Part model, mm, in its own coordinate system. Face numbers are marked on the shaded views. A direction names the side the tool comes from. Coordinates: 2 decimals unless noted, no trailing zeros. Order: outer loops, then holes, each group sorted by start corner. A loop starts at its lowest first (then second) coordinate and runs counter-clockwise, first axis right, second up.
from build123d import *

# Parameters (mm, degrees)
SKICA1_R                 = 45
P_IDAT_VYSUNUT_M1_DEPTH  = 10
SKICA3_R                 = 5
ODEBRAT_VYSUNUT_M1_DEPTH = 65.420493634
KRUHOV_POLE1_COUNT       = 4
SKICA4_R                 = 20
P_IDAT_VYSUNUT_M2_DEPTH  = 50
SKICA5_R                 = 10
ODEBRAT_VYSUNUT_M2_DEPTH = 81.932070281
ZAOBLIT1_R               = 5
ZKOSEN_1_SIZE            = 5


with BuildPart() as part:
    # Skica1 → Přidat vysunutím1 (new body)
    with BuildSketch(Plane(origin=(0, 0, 0), x_dir=(1, 0, 0), z_dir=(0, 1, 0))):
        with Locations(Location((0, 0, 0), (0, 0, 270))):
            Circle(SKICA1_R)
    extrude(amount=P_IDAT_VYSUNUT_M1_DEPTH)

    # Skica3 → Odebrat vysunutím1 (cut, through all)
    with BuildSketch(Plane(origin=(0, 10, 0), x_dir=(1, 0, 0), z_dir=(0, 1, 0))):
        with Locations(Location((0, 35, 0), (0, 0, 270))):
            Circle(SKICA3_R)
    odebrat_vysunut_m1 = extrude(amount=-ODEBRAT_VYSUNUT_M1_DEPTH, mode=Mode.SUBTRACT)

    # Kruhové pole1: Odebrat vysunutím1 ×4 about axis
    kruhov_pole1_axis = Axis((0, 0, 0), (0, 1, 0))
    for i in range(1, KRUHOV_POLE1_COUNT):
        add(odebrat_vysunut_m1.rotate(kruhov_pole1_axis, i * 360 / KRUHOV_POLE1_COUNT), mode=Mode.SUBTRACT)

    # Skica4 → Přidat vysunutím2 (add)
    with BuildSketch(Plane(origin=(0, 10, 0), x_dir=(1, 0, 0), z_dir=(0, 1, 0))):
        with Locations(Location((0, 0, 0), (0, 0, 270))):
            Circle(SKICA4_R)
    extrude(amount=-P_IDAT_VYSUNUT_M2_DEPTH)

    # Skica5 → Odebrat vysunutím2 (cut, through all)
    with BuildSketch(Plane.XZ.offset(40)):
        with Locations(Location((0, 0, 0), (0, 0, 270))):
            Circle(SKICA5_R)
    extrude(amount=-ODEBRAT_VYSUNUT_M2_DEPTH, mode=Mode.SUBTRACT)

    # Zaoblit1
    zaoblit1_edges = [part.edges().sort_by_distance(p)[0] for p in [
        (0, 0, -20),
    ]]
    fillet(zaoblit1_edges, radius=ZAOBLIT1_R)

    # Zkosení1
    zkosen_1_edges = [part.edges().sort_by_distance(p)[0] for p in [
        (0, -40, -20),
    ]]
    chamfer(zkosen_1_edges, length=ZKOSEN_1_SIZE)


solid = part.part
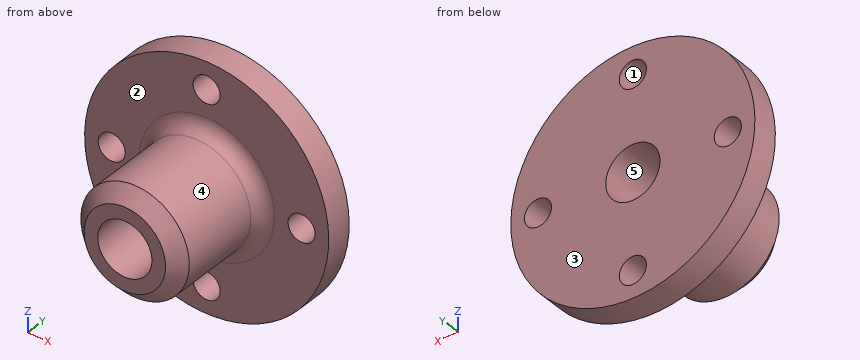
Q1. Which spindle directions (+Z, -Z, +X, -X, +Y, -Y) get a long thin tool onto all of the face, cutting with end or side? Do the marked faces 1 and 2. Say none if no direction does.
Results list:
face 1: +Y, -Y
face 2: -Y
Q2. Cut at B-B on z = 0. Write the cut outline in (x, y), and give its area (3 significant figures).
Results list:
outline: (-45, 0) - (-40, 0) - (-40, 10) - (-45, 10) - close; (-30, 0) - (-25, 0) arc R5 cw to (-20, -5) - (-20, -35) - (-15, -40) - (-10, -40) - (-10, 10) - (-30, 10) - close; (10, -40) - (15, -40) - (20, -35) - (20, -5) arc R5 cw to (25, 0) - (30, 0) - (30, 10) - (10, 10) - close; (40, 0) - (45, 0) - (45, 10) - (40, 10) - close
area: 1,290 mm2
Q3. Wall check: line 1 along X through (y, z) = (-27, 0); line 2 along Z through (x, y) = (0.5, -20); line 3 along Y through (x, z) = (27.5, -26.5). Give the ranges that are in metal, low to high.
Results list:
line 1: x = -20 to -10, 10 to 20
line 2: z = -19.99 to -9.99, 9.99 to 19.99
line 3: y = 0 to 10
Q4. Cut at C-C on z = 35. Write the cut outline in (x, y), and give its area (3 significant figures).
Results list:
outline: (-28.28, 0) - (-5, 0) - (-5, 10) - (-28.28, 10) - close; (5, 0) - (28.28, 0) - (28.28, 10) - (5, 10) - close
area: 466 mm2
Q5. Mould opens along Z. For the marked faces 3, 4 and 5 say: pulls with the +Z half, pulls with the -Z half, needs draft (parallel to the pull), parting line crosses it, or undercut.
Results list:
face 3: needs draft
face 4: parting line crosses it
face 5: undercut
Q6. Cut at A-A on x = 0. Write the cut outline in (y, z).
Results list:
outline: (-40, -15) - (-35, -20) - (-5, -20) arc R5 cw to (0, -25) - (0, -30) - (10, -30) - (10, -10) - (-40, -10) - close; (-40, 10) - (10, 10) - (10, 30) - (0, 30) - (0, 25) arc R5 cw to (-5, 20) - (-35, 20) - (-40, 15) - close; (0, -45) - (10, -45) - (10, -40) - (0, -40) - close; (0, 40) - (10, 40) - (10, 45) - (0, 45) - close
Q7. Pin check, flat tips, straight feed: pin 1 Ø6 at (x, y) = (-10, -13) entering from +Z (3 decimals); pin 2 Ø3 at (x, y) = (-19, 0.5) entering from +Z; pin 3 Ø8 at (y, z) = (-20.5, -0.5) entering from +X; pin 4 Ø9 at (x, z) = (-35, 0) entering from +Y. Stop position of each tip, or through.
Results list:
pin 1: stops at z = 18.735
pin 2: stops at z = 41.46
pin 3: stops at x = 20
pin 4: passes through
Q8. Cut at D-D on y = -22.5. Write the cut outline in (x, z).
Results list:
outline: circle Ø40 at (0, 0); hole circle Ø20 at (0, 0)
